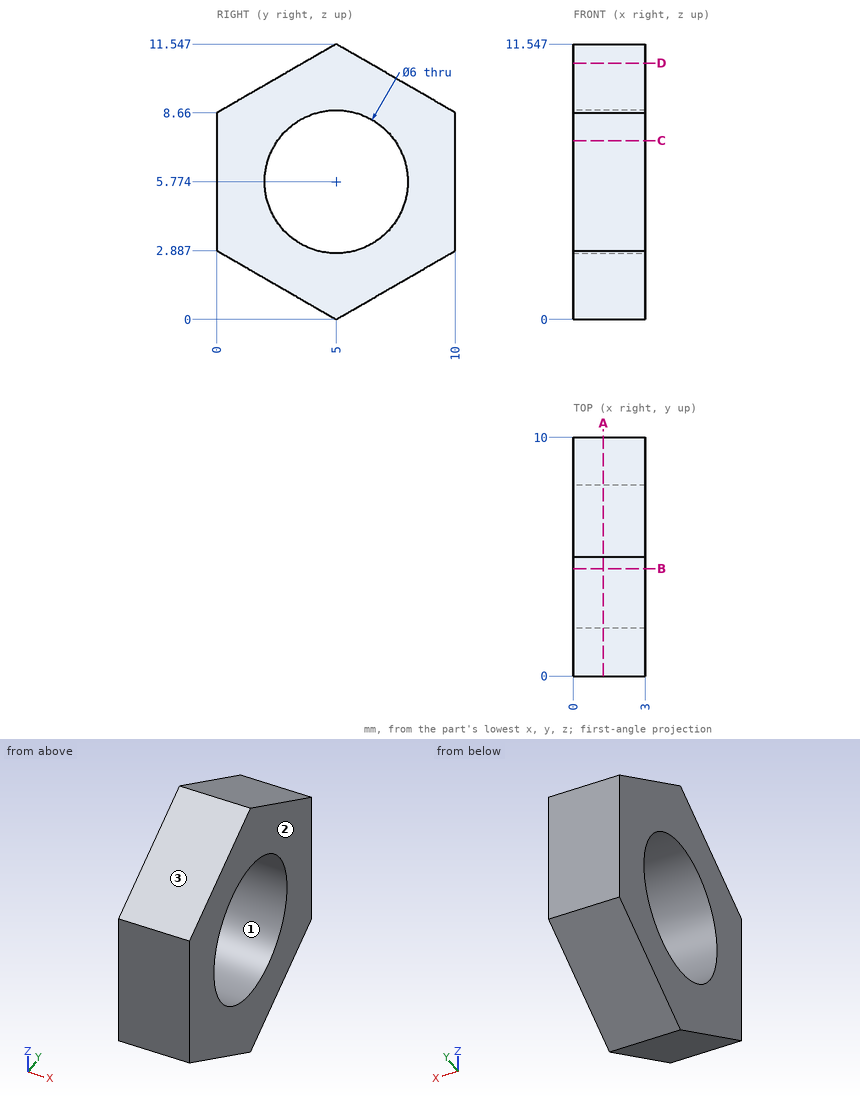
Verification items for this drawing (mm, ordinates from the low corner). Coordinates: 2 decimals unless noted, no trailing zeros. Order: outer loops, then holes, each group sorted by start corner. A loop starts at its lowest first (then second) coordinate and runs counter-clockwise, first axis right, second up.
Q1. Sectioned sample at A-A on x = 1.25. Record the cut outline in (y, z).
Reply:
outline: (0, 2.89) - (5, 0) - (10, 2.89) - (10, 8.66) - (5, 11.55) - (0, 8.66) - close; hole circle Ø6 at (5, 5.77)
Q2. Thickness scan on probe 1 along Z at (x, y) = (0.75, 7.75) (1 decimal); probe 2 along Y at (x, z) = (1.7, 7.25); probe 3 along Z at (x, y) = (1.1, 5.75) (1 decimal). Record the ranges inside material, lowest first.
Reply:
probe 1: z = 1.6 to 4.6, 7 to 10
probe 2: y = 0 to 2.39, 7.61 to 10
probe 3: z = 0.4 to 2.9, 8.7 to 11.1
Q3. Draft check along Z on the marked faces 1, 2 and 3. Enter one of: released by +Z, released by -Z, zero draft, split by the parting line, or undercut.
Reply:
face 1: undercut
face 2: zero draft
face 3: released by +Z
Q4. Sectioned sample at C-C on z = 7.5. Record the cut outline in (x, y).
Reply:
outline: (0, 0) - (3, 0) - (3, 2.55) - (0, 2.55) - close; (0, 7.45) - (3, 7.45) - (3, 10) - (0, 10) - close
Q5. Depth check by flat-ended pin: pin 1 Ø1 at (x, y) = (1.5, 4) entering from -Z; pin 2 Ø1 at (x, y) = (2.5, 1.5) entering from +Z (1 decimal). Enter the tip coordinate at first touch or a pass-through.
Reply:
pin 1: stops at z = 0.29
pin 2: stops at z = 9.8
Q6. Sectioned sample at D-D on z = 10.75. Record the cut outline in (x, y).
Reply:
outline: (0, 3.62) - (3, 3.62) - (3, 6.38) - (0, 6.38) - close
Q7. Sectioned sample at B-B on y = 4.5. Record the cut outline in (x, z) (1 decimal).
Reply:
outline: (0, 0.3) - (3, 0.3) - (3, 2.8) - (0, 2.8) - close; (0, 8.7) - (3, 8.7) - (3, 11.3) - (0, 11.3) - close
